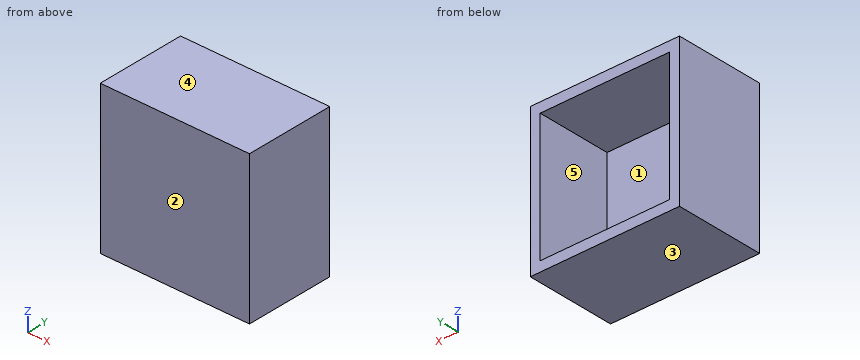
Autodesk Inventor part; units mm, degrees
ref_plane "YZ Plane" through (0, 0, 0) normal (1, 0, 0) x (0, 1, 0)
ref_plane "XZ Plane" through (0, 0, 0) normal (0, 1, 0) x (-1, 0, 0)
ref_plane "XY Plane" through (0, 0, 0) normal (0, 0, 1) x (1, 0, 0)
sketch "Sketch1" plane through (0, 0, 0) normal (0, 1, 0) x (-1, 0, 0)
  line L0 (0, 0) -> (30, 0)
  line L1 (30, 0) -> (30, -30)
  line L2 (30, -30) -> (0, -30)
  line L3 (0, -30) -> (0, 0)
  line L4 (28, -2) -> (2, -2)
  line L5 (2, -2) -> (2, -28)
  line L6 (2, -28) -> (28, -28)
  line L7 (28, -28) -> (28, -2)
  point P0 (0, -15)
  point P1 (2, -15)
  dimension "d0" = 30
  dimension "d1" = 30
  dimension "d2" = 2
  dimension "d3" = 2
  dimension "d4" = 2
  dimension "d5" = 2
extrude "Extrusion1" add sketch "Sketch1" along normal blind 15
sketch "Sketch2" plane through (0, 0, 0) normal (0, -1, 0) x (1, 0, 0)
  line L0 (-30, 0) -> (0, 0)
  line L1 (0, -30) -> (-30, -30)
  line L2 (-30, 0) -> (0, 0)
  line L3 (0, 0) -> (0, -30)
  line L4 (0, -30) -> (-30, -30)
  line L5 (-30, -30) -> (-30, 0)
extrude "Extrusion2" add sketch "Sketch2" along normal blind 3
properties part number "Boks_3DPrint"
CAD build for the part. Positions are in the model's coordinates, mm. Face numbers are marked on the shaded views. A direction names the side the tool comes from. Round coordinates to 2 decimals unless told otherwise and drop trailing zeros. Order: outer loops, then holes, each group sorted by start corner. A loop starts at its lowest first (then second) coordinate and runs counter-clockwise, first axis right, second up.
Item 1: Saw through at C-C on z = -4. Write the cut outline in (x, y).
Item 2: Mould opens along Z. For the marked faces 3, 4 and 5 say: pulls with the +Z half, pulls with the -Z half, needs draft (parallel to the pull), parting line crosses it, or undercut.
Item 3: Tool access for the marked faces 1 and 2: list every direction of +Z, -Z, +X, -X, +Y, -Y with a clear straight run to the whole face (end or side of a thin tool).
Item 4: Saw through at A-A on y = 11. Write the cut outline in (x, z).
Item 5: Saw through at B-B on x = -18.5. Write the cut outline in (y, z).
Item 6: Pin check, flat tips, straight feed: pin 1 (13 mm diameter, centred on x = -19.5, z = -16, fed in from +Y); pin 2 (10 mm diameter, centred on y = 8.5, z = -5.5, fed in from +X). Stop position of each tip, or through.
Item 7: Probe line 1 along Z through (x, y) = (-10, 4.75); line 2 along Y through (x, z) = (-12, -5). List the from-to ranges inside material, lowest first.
Reported:
1. outline: (-30, -3) - (0, -3) - (0, 15) - (-2, 15) - (-2, 0) - (-28, 0) - (-28, 15) - (-30, 15) - close
2. face 3: pulls with the -Z half
2. face 4: pulls with the +Z half
2. face 5: undercut
3. face 1: +Y
3. face 2: +Z, -Z, +X, -X, -Y
4. outline: (-30, -30) - (0, -30) - (0, 0) - (-30, 0) - close; hole (-28, -28) - (-2, -28) - (-2, -2) - (-28, -2) - close
5. outline: (-3, -30) - (15, -30) - (15, -28) - (0, -28) - (0, -2) - (15, -2) - (15, 0) - (-3, 0) - close
6. pin 1: stops at y = 0
6. pin 2: stops at x = 0
7. line 1: z = -30 to -28, -2 to 0
7. line 2: y = -3 to 0
